```python
from build123d import *

# Parameters (mm, degrees)
SKETCH1_W           = 50.8
SKETCH1_H           = 19.05
SKETCH1_R           = 6.35
BOSS_EXTRUDE1_DEPTH = 19.05
SKETCH2_R           = 8.73125
CUT_EXTRUDE1_DEPTH  = 1.5875
SKETCH3_R           = 3.175
CUT_EXTRUDE2_DEPTH  = 22.4155
SKETCH4_R           = 4.7625
CUT_EXTRUDE3_DEPTH  = 6.35


with BuildPart() as part:
    # Sketch1 → Boss-Extrude1 (new body)
    with BuildSketch(Plane.XY):
        Rectangle(SKETCH1_W, SKETCH1_H)
        Circle(SKETCH1_R, mode=Mode.SUBTRACT)
    extrude(amount=BOSS_EXTRUDE1_DEPTH)

    # Sketch2 → Cut-Extrude1 (cut)
    with BuildSketch(Plane.XY.offset(19.05)):
        Circle(SKETCH2_R)
    extrude(amount=-CUT_EXTRUDE1_DEPTH, mode=Mode.SUBTRACT)

    # Sketch3 → Cut-Extrude2 (cut)
    with BuildSketch(Plane.XZ.offset(9.525)):
        with Locations((-15.875, 9.525)):
            Circle(SKETCH3_R)
        with Locations((15.875, 9.525)):
            Circle(SKETCH3_R)
    extrude(amount=-CUT_EXTRUDE2_DEPTH, mode=Mode.SUBTRACT)

    # Sketch4 → Cut-Extrude3 (cut)
    with BuildSketch(Plane.XZ.offset(9.525)):
        with Locations((-15.875, 9.525)):
            Circle(SKETCH4_R)
        with Locations((15.875, 9.525)):
            Circle(SKETCH4_R)
    extrude(amount=-CUT_EXTRUDE3_DEPTH, mode=Mode.SUBTRACT)


solid = part.part
```
Build history of the part. All positions in model axes, mm. A direction names the side the tool comes from. Coordinates: 2 decimals unless noted, no trailing zeros. Order: outer loops, then holes, each group sorted by start corner. A loop starts at its lowest first (then second) coordinate and runs counter-clockwise, first axis right, second up. Notation, with made-up numbers: M 44.5,15.5 L 93.5,15.5 A22 cw 93.5,23.5 Z; hole C -12.5,54.5 d11. An arc over 180 degrees is marked long. One line per question, with ' | ' between items. Start each with the question number.
1. Wall check: line 1 along X through (y, z) = (-6.75, 13.5); line 2 along Y through (x, z) = (0, 8.75) (3 decimals); line 3 along X through (y, z) = (-4, 8.5). Give the ranges that are in metal, low to high. Write a range as [from, to].
2. Cut at B-B (z = 11.75). Write the cut outline in (x, y) (3 decimals), plus the area to 3 significant figures.
3. Flat gauge pins, fed straight in: P1, Ø7.5, axis at x = -15.875, z = 9.525, coming from the -Y side (3 decimals); P2, Ø5, axis at x = 3, y = 5, coming from the +Z side. Where does each tip first touch, or does it go through?
4. Tool access for faces 4 (the face through (-6, -3, 17.463)), 5 (the face through (0, 9.525, 9)), 6 (the face through (-15, -3.175, 6)): list every direction of +Z, -Z, +X, -X, +Y, -Y with a clear straight run to the whole face (end or side of a thin tool).
5. Cut at A-A (y = 5.5). Count the separate pieces of the cut face and the enclosed holes in it, plus the area to 3 significant figures.
6. Mould opens along Z. For faces 1 (the face through (17, -3.175, 6)), 2 (the face through (25.4, 0, 9)), 3 (the face through (-6, 9, 19.05)) say: +Z half, -Z half, draft (parallel to the pull), parting line (faces both ways), or undercut.
The answers:
1) line 1: x = [-25.4, -18.5], [-13.25, 13.25], [18.5, 25.4] | line 2: y = [-9.525, -6.35], [6.35, 9.525] | line 3: x = [-25.4, -20.53], [-11.22, -4.93], [4.93, 11.22], [20.53, 25.4]
2) outline: M -25.4,-9.525 L -20.086,-9.525 L -20.086,-3.175 L -18.14,-3.175 L -18.14,9.525 L -25.4,9.525 Z; M -13.61,-3.175 L -11.664,-3.175 L -11.664,-9.525 L 11.664,-9.525 L 11.664,-3.175 L 13.61,-3.175 L 13.61,9.525 L -13.61,9.525 Z; M 18.14,-3.175 L 20.086,-3.175 L 20.086,-9.525 L 25.4,-9.525 L 25.4,9.525 L 18.14,9.525 Z; hole C 0,0 d12.7 | area: 619 mm2
3) P1: stops at y = -3.175 | P2: stops at z = 17.46
4) face 4: +Z | face 5: +Z, -Z, +X, -X, +Y | face 6: -Y
5) separate pieces: 2 | enclosed holes: 2 | area: 772 mm2
6) face 1: undercut | face 2: draft | face 3: +Z half
